from build123d import *

# Parameters (mm, degrees)
BASE_FLANGE1_DEPTH = 16
SKETCH3_R          = 11
CUT_HOLES_DEPTH    = 1042.876868884


# Sheet-metal steps are written as plain solids
with BuildPart() as part:
    # Sketch1 → Base-Flange1 (new body)
    with BuildSketch(Plane(origin=(0, 0, 0), x_dir=(0, 0, -1), z_dir=(1, 0, 0))):
        with BuildLine():
            Line((305.218612063, 670.218640107), (400.630345104, 785.962327615))
            ThreePointArc((400.630345104, 785.962327615), (416.512049286, 798.70874281), (436.159147295, 804.065156521))
            Line((436.159147295, 804.065156521), (574.750134607, 812.541744435))
            ThreePointArc((574.750134607, 812.541744435), (615.094497482, 808.133571726), (651.662136675, 790.529385681))
            Line((651.662136675, 790.529385681), (0, 0))
            Line((0, 0), (-140, 0))
            Line((-140, 0), (-140, 94.22160699))
            ThreePointArc((-140, 94.22160699), (-134.117601526, 128.01327879), (-117.162458339, 157.829429018))
            Line((-117.162458339, 157.829429018), (-89.113742378, 191.855242319))
            ThreePointArc((-89.113742378, 191.855242319), (127.343049427, 415.134985706), (305.218612063, 670.218640107))
        make_face()
    extrude(amount=-BASE_FLANGE1_DEPTH)

    # Sketch3 → Cut-Holes (cut, through all)
    with BuildSketch(Plane(origin=(0, 0, 0), x_dir=(0, 0, -1), z_dir=(1, 0, 0))):
        with Locations((-40.344519187, 192.562071849)):
            Circle(SKETCH3_R)
        with Locations((-102.086703913, 106.4)):
            Circle(SKETCH3_R)
        with Locations((-9.1, 98.818911988)):
            Circle(SKETCH3_R)
        with Locations((37.497875264, 163.846890742)):
            Circle(SKETCH3_R)
    extrude(amount=-CUT_HOLES_DEPTH, mode=Mode.SUBTRACT)


solid = part.part
Design review of the part built by this model. Coordinates are the model's own, in mm. Coordinates: 2 decimals unless noted, no trailing zeros. Order: outer loops, then holes, each group sorted by start corner. A loop starts at its lowest first (then second) coordinate and runs counter-clockwise, first axis right, second up. Notation, with made-up numbers: M -11,80 L -7,80 A10 cw -7,86 Z; hole C 38,49 d3. An arc over 180 degrees is marked long. Use a Markdown table: item, result.
(1) Add section C-C (y = 647). Give the boundary of the cut face in (x, z), then the cut area to 3 significant figures.
Worked answers:
| item | result |
|---|---|
| outline | M -16,-533.35 L 0,-533.35 L 0,-291.44 L -16,-291.44 Z |
| area | 3,870 mm2 |
(2) Add section B-B (z = 9.1). Give the boundary of the cut face in (x, y).
Worked answers:
| item | result |
|---|---|
| outline | M -16,0 L 0,0 L 0,87.82 L -16,87.82 Z; M -16,109.82 L 0,109.82 L 0,266.2 L -16,266.2 Z |
(3) For P1, Ø8, axis at x = -7, z = -14, coming from the -Y side; P2, Ø20, axis at y = 98.82, z = 9.1, coming from the -X side; P3, Ø3, axis at x = -8, y = 232, coming from the -Z side; P4, Ø8, axis at x = -4.5, y = 443, coming from the +Z side, all flat-tipped, find the tip position at first contact; note any pin that passes through.
Worked answers:
| item | result |
|---|---|
| P1 | stops at y = 12.13 |
| P2 | passes through |
| P3 | stops at z = -192.48 |
| P4 | stops at z = -146.7 |
(4) Add section D-D (z = -505.5). Give the boundary of the cut face in (x, y).
Worked answers:
| item | result |
|---|---|
| outline | M -16,613.22 L 0,613.22 L 0,808.31 L -16,808.31 Z |
(5) Draft analysis for pull direction Y (two halves, no side actions). For faces 1 (the cylindrical face through (-7.89, 153.11, -35.11)), 2 (the flat face through (-7.888, 400.798, -330.393)), 3 (the cylindrical face through (-7.89, 127.56, 134.28)), 4 (the cylindrical face through (-7.888, 181.824, 42.729)), state which applies: released by +Y, released by -Y, zero draft, split by the parting line, or undercut.
Worked answers:
| item | result |
|---|---|
| face 1 | undercut |
| face 2 | released by -Y |
| face 3 | released by +Y |
| face 4 | undercut |
(6) Wall thickness on probe 1 along Y at (x, z) = (-4.5, 41); probe 2 along Z at (x, y) = (-2.5, 383.5); probe 3 along Y at (x, z) = (-7.25, -269): over which ranges is each line inside the solid? List them lowest first.
Worked answers:
| item | result |
|---|---|
| probe 1 | y = 0 to 181.58, 203.54 to 235.54 |
| probe 2 | z = -316.13 to -100.69 |
| probe 3 | y = 326.32 to 610.67 |
(7) Add section A-A (x = -6.5). Give the boundary of the cut face in (y, z), then the cut area to 3 significant figures.
Worked answers:
| item | result |
|---|---|
| outline | M 0,0 L 790.53,-651.66 A120 ccw 812.54,-574.75 L 804.07,-436.16 A50 ccw 785.96,-400.63 L 670.22,-305.22 A1934.15 cw 191.86,89.11 L 157.83,117.16 A100 ccw 94.22,140 L 0,140 Z; hole C 98.82,9.1 d22; hole C 106.4,102.09 d22; hole C 163.85,-37.5 d22; hole C 192.56,40.34 d22 |
| area | 180,000 mm2 |
